Verification items for the finished model (mm, model axes). A direction names the side the tool comes from. Give positions to 0.01 mm unless a question says otherwise; leave off trailing zeros. Order: outer loops, then holes, each group sorted by start corner. A loop starts at its lowest first (then second) coordinate and runs counter-clockwise, first axis right, second up.
(1) Scan lines: L1, parallel to Y at x = -18, z = 27.5; L2, parallel to Y at x = -10.25, z = 32.5; L3, parallel to Z at x = -13.75, y = -25.25. Record each from-to range of solid material in increasing order.
(2) Sectioned sample at B-B on z = 6.5. Record the cut outline in (x, y).
(3) Mould release check, pull along Z, two halves, no side actions. Record for faces 5 (the face through (-13.3, -18.2, 30)), 6 (the face through (-16.513, -24.136, 17.686)), 7 (the face through (-20, -24, 0)): pulls with the +Z half, pulls with the -Z half, needs draft (parallel to the pull), parting line crosses it, or undercut.
(4) Access from +Z, -Z, +X, -X, +Y, -Y to the whole of each face (thin tool, end or side, straight path). Record for faces 1 (the face through (-23.92, -24.186, 34.624)), 2 (the face through (-13, -30.032, 10)), 3 (the face through (-23, -20, 29.5)), 4 (the face through (-15, -26.762, 30)).
(5) Sectioned sample at C-C on z = 14. Record the cut outline in (x, y).
(6) Sectioned sample at A-A on z = 32. Record the cut outline in (x, y).
(7) Gauge pin test, flat ends, axial feed: pin 1 (12 mm diameter, centred on x = -20, z = 8, fed in from +Y); pin 2 (2 mm diameter, centred on x = -7.5, y = -19.5, fed in from -Z); pin 3 (2.5 mm diameter, centred on x = -8.45, y = -24.07, fed in from -Z); pin 4 (1 mm diameter, centred on x = -23.5, y = -28.5, fed in from +Z). Record the tip position at first contact, or that the pin passes through.
(8) Sectioned sample at D-D on x = -5. Record the cut outline in (y, z).
```python
from build123d import *

# Parameters (mm, degrees)
SKETCH1_W               = 22.054431489
SKETCH1_H               = 12.5
BOSS_EXTRUDE1_DEPTH     = 40
CUT_EXTRUDE1_DEPTH      = 10
CUT_EXTRUDE1_DEPTH_BACK = 15
SKETCH2_R               = 1.5
FILLET3_R               = 2
SKETCH5_R               = 1.5
CUT_EXTRUDE4_DEPTH      = 53.86644408
SKETCH16_W              = 22.16406654
SKETCH16_H              = 3.097743049
SKETCH16_W_2            = 22.194630718
SKETCH16_H_2            = 2.724396189
CUT_EXTRUDE6_DEPTH      = 8.5
FILLET4_R               = 2
SKETCH17_W              = 17.85596127
SKETCH17_H              = 3.097743049
SKETCH17_H_2            = 2.724396189
CUT_EXTRUDE7_DEPTH      = 5
SKETCH18_W              = 23.758682738
SKETCH18_H              = 0.759330362
SKETCH18_W_2            = 23.717859304
SKETCH18_H_2            = 0.728261761
CUT_EXTRUDE8_DEPTH      = 20


with BuildPart() as part:
    # Sketch1 → Boss-Extrude1 (new body)
    with BuildSketch(Plane.XY):
        with Locations((-13.228930986, -24.070183414)):
            Rectangle(SKETCH1_W, SKETCH1_H)
    extrude(amount=BOSS_EXTRUDE1_DEPTH)

    # Sketch2 → Cut-Extrude1 (cut, two sides: drawn at the far end of the back side and taken through both)
    with BuildSketch(Plane.XZ.offset(30.320183414).offset(-CUT_EXTRUDE1_DEPTH_BACK)):
        with Locations(Location((-13.228930986, 6.5, 0), (0, 0, 90))):
            Circle(SKETCH2_R)
        with Locations(Location((-13.228930986, 31.5, 0), (0, 0, 90))):
            Circle(SKETCH2_R)
        with BuildLine():
            Line((-4.478930986, 29.25), (-2.201715242, 29.25))
            add(Edge.make_bspline(
                [(-24.256146731, 29.25), (-34.277912729, 38.417119108), (-13.227499763, 50.308047167), (7.840407292, 38.416977249), (-2.201715242, 29.25)],
                knots=[0, 0, 0, 0, 0.49986218, 1, 1, 1, 1], degree=3))
            add(Edge.make_bspline(
                [(-6.103895584, 34.329012749), (-10.720559386, 33.527203043), (-28.641384523, 40.845191705), (-24.256146731, 29.25)],
                knots=[0, 0, 0, 0, 1, 1, 1, 1], degree=3))
            ThreePointArc((-6.103895584, 34.329012749), (-4.895067543, 31.916312081), (-4.478930986, 29.25))
        make_face()
        with BuildLine():
            Line((-4.478930986, 8.75), (-2.201715242, 8.75))
            add(Edge.make_bspline(
                [(-2.201715242, 8.75), (5.39210746, 3.880294823), (-0.777052631, -4.523329032), (-17.174300591, -10.623347238), (-34.821400648, -0.026005424), (-24.256146731, 8.75)],
                knots=[0, 0, 0, 0, 0.283272691, 0.504244858, 1, 1, 1, 1], degree=3))
            add(Edge.make_bspline(
                [(-23.490579314, 0), (-24.966512963, 4.237786421), (-24.256146731, 8.75)],
                knots=[0, 0, 0, 1, 1, 1], degree=2))
            Line((-23.490579314, 0), (-13.228930986, 0))
            ThreePointArc((-13.228930986, 0), (-7.041746651, 2.562815665), (-4.478930986, 8.75))
        make_face()
    extrude(amount=CUT_EXTRUDE1_DEPTH + CUT_EXTRUDE1_DEPTH_BACK, mode=Mode.SUBTRACT)

    # Fillet3
    # the kernel refuses this fillet: 2 mm, written as the material it takes off along each edge
    with BuildSketch(Plane(origin=(-24.256146731, -17.820183414, -5.498495188), x_dir=(1, 0, 0), z_dir=(0, 0, 1))) as fillet3_piece_1:
        with BuildLine():
            CenterArc((FILLET3_R, -FILLET3_R), FILLET3_R, 90, 90)
            Line((0, -FILLET3_R), (-FILLET3_R * 0.02, -FILLET3_R))
            Line((-FILLET3_R * 0.02, -FILLET3_R), (-FILLET3_R * 0.02, FILLET3_R * 0.02))
            Line((-FILLET3_R * 0.02, FILLET3_R * 0.02), (FILLET3_R, FILLET3_R * 0.02))
            Line((FILLET3_R, FILLET3_R * 0.02), (FILLET3_R, 0))
        make_face()
    extrude(amount=44.984872581, mode=Mode.SUBTRACT)
    with BuildSketch(Plane(origin=(-24.256146731, -30.320183414, -5.498495188), x_dir=(1, 0, 0), z_dir=(0, 0, 1))) as fillet3_piece_2:
        with BuildLine():
            CenterArc((FILLET3_R, FILLET3_R), FILLET3_R, 180, 90)
            Line((0, FILLET3_R), (-FILLET3_R * 0.02, FILLET3_R))
            Line((-FILLET3_R * 0.02, FILLET3_R), (-FILLET3_R * 0.02, -FILLET3_R * 0.02))
            Line((-FILLET3_R * 0.02, -FILLET3_R * 0.02), (FILLET3_R, -FILLET3_R * 0.02))
            Line((FILLET3_R, -FILLET3_R * 0.02), (FILLET3_R, 0))
        make_face()
    extrude(amount=44.984872581, mode=Mode.SUBTRACT)
    with BuildSketch(Plane(origin=(-24.256146731, -17.374523396, 3.001504812), x_dir=(0.16676818592575848, -1.2260366807919533e-15, -0.9859961319209278), z_dir=(0, -1, 0))) as fillet3_piece_3:
        with BuildLine():
            CenterArc((0.168096911, 1.999974157), FILLET3_R, 260.400032587, 9.891234523)
            Line((-0.165439461, 0.027981894), (-0.172110188, -0.011457952))
            Line((-0.172110188, -0.011457952), (-0.006670727, -0.039439845))
            Line((-0.006670727, -0.039439845), (-0.00020343, -0.039999483))
            ThreePointArc((-0.00020343, -0.039999483), (0.089132026, -0.040226606), (0.178467349, -0.039999483))
            Line((0.178467349, -0.039999483), (0.178264007, 0))
        make_face()
    extrude(amount=13.391320036, mode=Mode.SUBTRACT)
    with BuildSketch(Plane(origin=(-24.256146731, -14.125185169, 34.486377393), x_dir=(0.8125654725304995, 0, 0.5828699279009736), z_dir=(0, -1, 0))) as fillet3_piece_4:
        with BuildLine():
            CenterArc((1.058597408, -1.955531144), FILLET3_R, 77.895172565, 66.452175148)
            Line((-0.566533537, -0.789791288), (-0.599036156, -0.766476491))
            Line((-0.599036156, -0.766476491), (-0.032502619, 0.023314797))
            Line((-0.032502619, 0.023314797), (-0.009827922, 0.038773856))
            ThreePointArc((-0.009827922, 0.038773856), (0.740246051, 0.125750941), (1.486387336, 0.039110623))
            Line((1.486387336, 0.039110623), (1.477999298, 0))
        make_face()
    extrude(amount=19.88999649, mode=Mode.SUBTRACT)

    # Sketch5 → Cut-Extrude4 (cut, through all)
    with BuildSketch(Plane.XY):
        with Locations(Location((-18.011106811, -24.070183414, 0), (0, 0, 180))):
            Circle(SKETCH5_R)
        with Locations(Location((-8.446755162, -24.070183414, 0), (0, 0, 180))):
            Circle(SKETCH5_R)
    extrude(amount=CUT_EXTRUDE4_DEPTH, mode=Mode.SUBTRACT)

    # Sketch16 → Cut-Extrude6 (cut)
    with BuildSketch(Plane.XY.offset(38)):
        with Locations((-13.228930985, -20.132105575)):
            Rectangle(SKETCH16_W, SKETCH16_H)
        with Locations((-13.228930985, -28.124114993)):
            Rectangle(SKETCH16_W_2, SKETCH16_H_2)
    extrude(amount=-CUT_EXTRUDE6_DEPTH, mode=Mode.SUBTRACT)

    # Fillet4
    # the kernel refuses this fillet: 2 mm, written as the material it takes off along each edge
    with BuildSketch(Plane(origin=(-6.103895584, -21.985936801, 34.329012749), x_dir=(0.5153680546007453, 0, -0.8569689424343471), z_dir=(0, 1, 0))) as fillet4_piece_1:
        with BuildLine():
            CenterArc((1.205528974, 1.993941708), FILLET4_R, 212.228268917, 62.232476225)
            Line((-0.486331325, 0.927354287), (-0.520168531, 0.906022538))
            ThreePointArc((-0.520168531, 0.906022538), (-0.25689069, 0.456334761), (-0.037300681, -0.01444504))
            Line((-0.037300681, -0.01444504), (-0.003111043, -0.039878834))
            ThreePointArc((-0.003111043, -0.039878834), (0.68054055, -0.066505026), (1.364192143, -0.039878834))
            Line((1.364192143, -0.039878834), (1.3610811, 0))
        make_face()
    extrude(amount=7.568456138, mode=Mode.SUBTRACT)
    with BuildSketch(Plane(origin=(-6.103895584, -30.164619649, 34.329012749), x_dir=(0.5153680546007453, 0, -0.8569689424343471), z_dir=(0, 1, 0))) as fillet4_piece_2:
        with BuildLine():
            CenterArc((1.205528974, 1.993941708), FILLET4_R, 212.228268917, 62.232476225)
            Line((-0.486331325, 0.927354287), (-0.520168531, 0.906022538))
            ThreePointArc((-0.520168531, 0.906022538), (-0.25689069, 0.456334761), (-0.037300681, -0.01444504))
            Line((-0.037300681, -0.01444504), (-0.003111043, -0.039878834))
            ThreePointArc((-0.003111043, -0.039878834), (0.68054055, -0.066505026), (1.364192143, -0.039878834))
            Line((1.364192143, -0.039878834), (1.3610811, 0))
        make_face()
    extrude(amount=11.886345299, mode=Mode.SUBTRACT)
    with BuildSketch(Plane(origin=(-6.103895584, -33.722886164, 34.329012749), x_dir=(0.5153680546007453, 0, -0.8569689424343471), z_dir=(0, 1, 0))) as fillet4_piece_3:
        with BuildLine():
            CenterArc((1.205528974, 1.993941708), FILLET4_R, 212.228268917, 62.232476225)
            Line((-0.486331325, 0.927354287), (-0.520168531, 0.906022538))
            ThreePointArc((-0.520168531, 0.906022538), (-0.25689069, 0.456334761), (-0.037300681, -0.01444504))
            Line((-0.037300681, -0.01444504), (-0.003111043, -0.039878834))
            ThreePointArc((-0.003111043, -0.039878834), (0.68054055, -0.066505026), (1.364192143, -0.039878834))
            Line((1.364192143, -0.039878834), (1.3610811, 0))
        make_face()
    extrude(amount=7.639275828, mode=Mode.SUBTRACT)

    # Sketch17 → Cut-Extrude7 (cut)
    with BuildSketch(Plane.XY.offset(29.5)):
        with Locations((-13.410483779, -20.132105575)):
            Rectangle(SKETCH17_W, SKETCH17_H)
        with Locations((-13.410483779, -28.124114993)):
            Rectangle(SKETCH17_W, SKETCH17_H_2)
    extrude(amount=-CUT_EXTRUDE7_DEPTH, mode=Mode.SUBTRACT)

    # Sketch18 → Cut-Extrude8 (cut)
    with BuildSketch(Plane.XY):
        with Locations((-13.209901434, -17.695854471)):
            Rectangle(SKETCH18_W, SKETCH18_H)
        with Locations((-13.189489717, -30.396128596)):
            Rectangle(SKETCH18_W_2, SKETCH18_H_2)
    extrude(amount=CUT_EXTRUDE8_DEPTH, mode=Mode.SUBTRACT)


solid = part.part
```
Ans:
1. L1: y = -30.32 to -29.49, -26.76 to -25.57, -22.57 to -21.68, -18.58 to -17.82
1. L2: y = -30.32 to -29.49, -26.76 to -21.68, -18.58 to -17.82
1. L3: z = 0 to 5.09, 7.91 to 30.09, 32.91 to 35.22
2. outline: (-24.26, -28.32) arc R2 ccw to (-23.29, -30.03) - (-14.73, -30.03) - (-14.73, -18.08) - (-23.23, -18.08) arc R2 ccw to (-24.26, -19.82) - close; (-11.73, -30.03) - (-4.77, -30.03) - (-4.77, -18.08) - (-11.73, -18.08) - close; hole circle Ø3 at (-18.01, -24.07); hole circle Ø3 at (-8.45, -24.07)
3. face 5: undercut
3. face 6: needs draft
3. face 7: pulls with the -Z half
4. face 1: +Z, -X, +Y, -Y
4. face 2: -Z, +X, -X, -Y
4. face 3: +Z, +X, -X
4. face 4: +Z
5. outline: (-24.26, -28.32) arc R2 ccw to (-23.29, -30.03) - (-2.2, -30.03) - (-2.2, -18.08) - (-23.23, -18.08) arc R2 ccw to (-24.26, -19.82) - close; hole circle Ø3 at (-18.01, -24.07); hole circle Ø3 at (-8.45, -24.07)
6. outline: (-24.26, -26.76) - (-14.64, -26.76) - (-14.64, -21.68) - (-24.26, -21.68) - close; (-23.88, -29.49) arc R2 ccw to (-22.26, -30.32) - (-14.64, -30.32) - (-14.64, -29.49) - close; (-23.83, -18.58) - (-14.64, -18.58) - (-14.64, -17.82) - (-22.26, -17.82) arc R2 ccw to start; (-11.81, -30.32) - (-4.92, -30.32) - (-4.92, -29.49) - (-11.81, -29.49) - close; (-11.81, -26.76) - (-4.92, -26.76) - (-4.92, -21.68) - (-11.81, -21.68) - close; (-11.81, -18.58) - (-4.92, -18.58) - (-4.92, -17.82) - (-11.81, -17.82) - close; hole circle Ø3 at (-18.01, -24.07); hole circle Ø3 at (-8.45, -24.07)
7. pin 1: stops at y = -18.08
7. pin 2: stops at z = 1.39
7. pin 3: passes through
7. pin 4: stops at z = 29.5
8. outline: (-30.32, 20) - (-30.03, 20) - (-30.03, 5.78) - (-18.08, 5.78) - (-18.08, 20) - (-17.82, 20) - (-17.82, 32.22) - (-18.58, 32.22) - (-18.58, 24.5) - (-21.68, 24.5) - (-21.68, 32.22) - (-26.76, 32.22) - (-26.76, 24.5) - (-29.49, 24.5) - (-29.49, 32.22) - (-30.32, 32.22) - close
